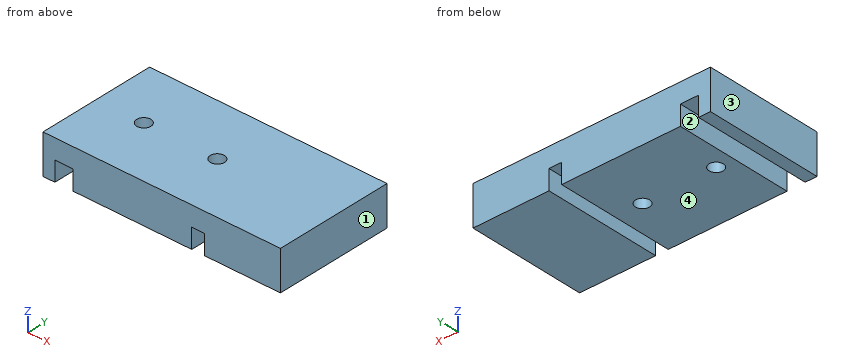
from build123d import *

# Parameters (mm, degrees)
F0_W     = 60
F0_H     = 30
F1_DEPTH = 5
F2_W     = 3.2
F2_H     = 30
F2_W_2   = 4.6
F3_DEPTH = 5
F4_R     = 1.8
F5_DEPTH = 26
F6_R     = 1.8
F7_DEPTH = 26


with BuildPart() as f1:
    # F0 (on Top) → F1 (new body, symmetric)
    with BuildSketch(Plane.XY):
        Rectangle(F0_W, F0_H)
    extrude(amount=F1_DEPTH, both=True)

    # F2 (on face) → F3 (cut)
    with BuildSketch(Plane(origin=(0, 0, -5), x_dir=(1, 0, 0), z_dir=(0, 0, -1))):
        with Locations((9.191833, 0)):
            Rectangle(F2_W, F2_H)
        with Locations((-24.708167, 0)):
            Rectangle(F2_W_2, F2_H)
    extrude(amount=-F3_DEPTH, mode=Mode.SUBTRACT)

    # F4 (on face) → F5 (cut)
    with BuildSketch(Plane.XY.offset(5)):
        with Locations((-17.986729, 0)):
            Circle(F4_R)
    extrude(amount=-F5_DEPTH, mode=Mode.SUBTRACT)

    # F6 (on face) → F7 (cut)
    with BuildSketch(Plane.XY.offset(5)):
        with Locations((0.613271, 0)):
            Circle(F6_R)
    extrude(amount=-F7_DEPTH, mode=Mode.SUBTRACT)


solid = f1.part
Design review of the part built by this model. Coordinates are the model's own, in mm. Face numbers are marked on the shaded views. Give positions to 0.01 mm unless a question says otherwise; leave off trailing zeros. Order: outer loops, then holes, each group sorted by start corner. A loop starts at its lowest first (then second) coordinate and runs counter-clockwise, first axis right, second up. Notation, with made-up numbers: (39.25, -3) - (43.25, -3) arc R31 cw to (43.25, 35) - close; hole circle Ø9 at (-21.5, 37.5). An arc over 180 degrees is marked (long way). Use CSV: the item, a comma, the result in double quotes. Start each with the question number.
Q1. Take a section at A-A (z = -1). State the section outline as (x, y) points, and give its area (3 significant figures).
Q2. Take a section at D-D (x = -26). State the section outline as (y, z) points, and give its area (3 significant figures).
Q3. Draft analysis for pull direction X (two halves, no side actions). For the marked faces 1, 2, 3 and 4, state which applies: pulls with the +X half, pulls with the -X half, needs draft (parallel to the pull), parting line crosses it, or undercut.
Q4. Take a section at C-C (y = -6.25). State the section outline as (x, z) points.
Q5. For line 1 (X direction, y = 5, z = -0.5); line 2 (X direction, y = -1.5, z = 4.25); line 3 (Z direction, x = 9, y = -2.5), list the stretches that pass through material, from the lowest coordinate up.
Q6. Take a section at B-B (y = 0). State the section outline as (x, z) points.
Q7. For P1, Ø1.6, axis at x = 8.5, y = -1, coming from the -Z side, flat-tipped, find the tip position at first contact; note if it passes through.
Calculated:
1,outline,"(-30, -15) - (-27.01, -15) - (-27.01, 15) - (-30, 15) - close; (-22.41, -15) - (7.59, -15) - (7.59, 15) - (-22.41, 15) - close; (10.79, -15) - (30, -15) - (30, 15) - (10.79, 15) - close; hole circle Ø3.6 at (-17.99, 0); hole circle Ø3.6 at (0.61, 0)"
1,area,"1,550 mm²"
2,outline,"(-15, 0) - (15, 0) - (15, 5) - (-15, 5) - close"
2,area,"150 mm²"
3,face 1,"pulls with the +X half"
3,face 2,"undercut"
3,face 3,"pulls with the -X half"
3,face 4,"needs draft"
4,outline,"(-30, -5) - (-27.01, -5) - (-27.01, 0) - (-22.41, 0) - (-22.41, -5) - (7.59, -5) - (7.59, 0) - (10.79, 0) - (10.79, -5) - (30, -5) - (30, 5) - (-30, 5) - close"
5,line 1,"x = -30 to -27.01, -22.41 to 7.59, 10.79 to 30"
5,line 2,"x = -30 to -18.98, -16.99 to -0.38, 1.61 to 30"
5,line 3,"z = 0 to 5"
6,outline,"(-30, -5) - (-27.01, -5) - (-27.01, 0) - (-22.41, 0) - (-22.41, -5) - (-19.79, -5) - (-19.79, 5) - (-30, 5) - close; (-16.19, -5) - (-1.19, -5) - (-1.19, 5) - (-16.19, 5) - close; (2.41, -5) - (7.59, -5) - (7.59, 0) - (10.79, 0) - (10.79, -5) - (30, -5) - (30, 5) - (2.41, 5) - close"
7,P1,"stops at z = 0"
